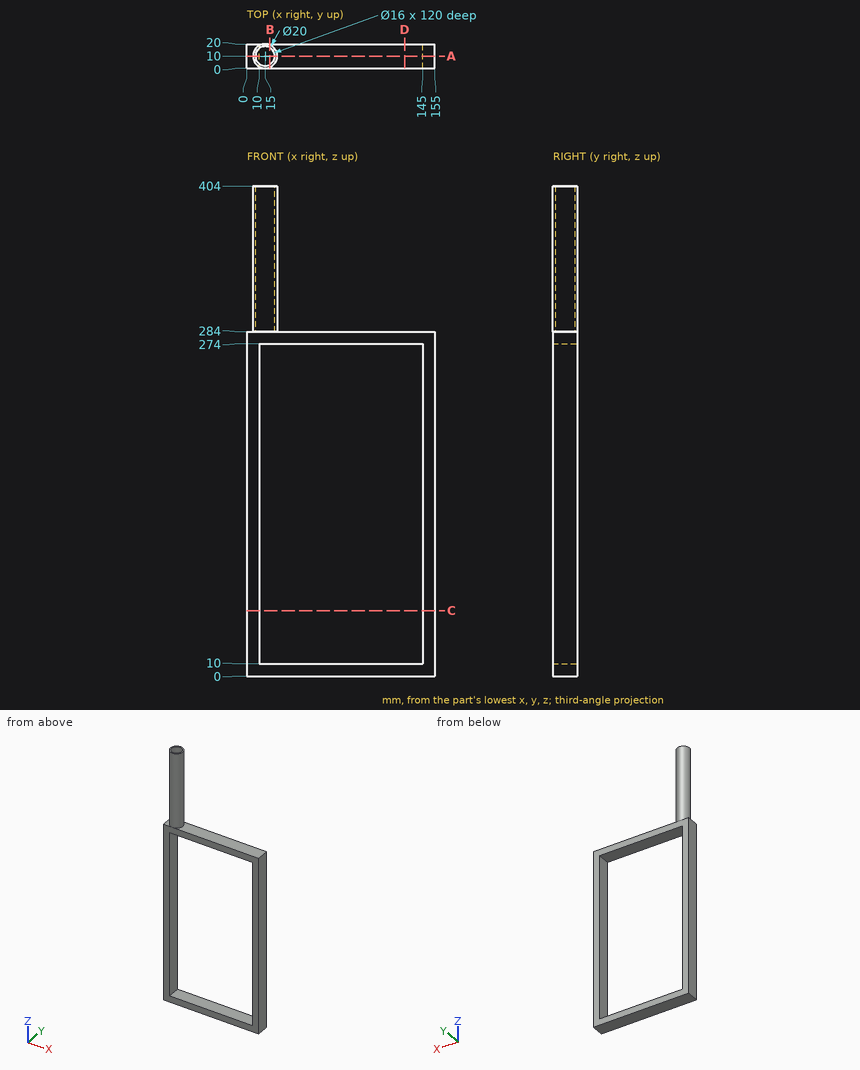
Drawing for the job (mm, zero at the part's lowest x, y, z). Round coordinates to 2 decimals unless told otherwise and drop trailing zeros. Loops run counter-clockwise (first coordinate to the right, second up) from the corner with the lowest first, then second, coordinate; pieces in that order, holes last. Notation, with made-up numbers: (-12.5, 26) - (2.5, 26) arc R18 cw to (2.5, 38) - close; hole circle Ø1 at (12, 66.5). An arc over 180 degrees is marked (long way). Return JSON: item names as keys, results as strings. Group by question number.
Q1. Drill centre lines: line 1 along Z through (x, y) = (98, 1); line 2 along X through (y, z) = (12.25, 79.5); line 3 along Z through (x, y) = (146, 11.5). Where is each one in solid material? Low to high. Write a range as [from, to].
Q2. Band-saw the part on D-D on x = 130. Give the cut face in (y, z), plus the area to 3 significant figures.
Q3. Band-saw the part on A-A on y = 10. Give the cut face in (x, z).
Q4. Flat gauge pin, fed straight in: pin 1 Ø8 at (x, y) = (68, 7) entering from +Z. Where does the tip first touch, or does it go through?
Q5. Band-saw the part on B-B on x = 19. Give the cut face in (y, z), plus the area to 3 significant figures.
Q6. Band-saw the part on C-C on z = 54. Give the cut face in (x, y).
Solutions:
{
 "1": {"line 1": "z = [0, 10], [274, 284]", "line 2": "x = [0, 10], [145, 155]", "line 3": "z = [0, 284]"},
 "2": {"outline": "(0, 0) - (20, 0) - (20, 10) - (0, 10) - close; (0, 274) - (20, 274) - (20, 284) - (0, 284) - close", "area": "400 mm^2"},
 "3": {"outline": "(0, 0) - (155, 0) - (155, 284) - (25, 284) - (25, 404) - (23, 404) - (23, 284) - (7, 284) - (7, 404) - (5, 404) - (5, 284) - (0, 284) - close; hole (10, 10) - (145, 10) - (145, 274) - (10, 274) - close"},
 "4": {"pin 1": "stops at z = 284"},
 "5": {"outline": "(0, 0) - (20, 0) - (20, 10) - (0, 10) - close; (0, 274) - (20, 274) - (20, 284) - (19.17, 284) - (19.17, 404) - (16.93, 404) - (16.93, 284) - (3.07, 284) - (3.07, 404) - (0.83, 404) - (0.83, 284) - (0, 284) - close", "area": "937 mm^2"},
 "6": {"outline": "(0, 0) - (10, 0) - (10, 20) - (0, 20) - close; (145, 0) - (155, 0) - (155, 20) - (145, 20) - close"}
}
